Design review of the part built by this model. Coordinates are the model's own, in mm. A direction names the side the tool comes from. Give positions to 0.01 mm unless a question says otherwise; leave off trailing zeros. Order: outer loops, then holes, each group sorted by start corner. A loop starts at its lowest first (then second) coordinate and runs counter-clockwise, first axis right, second up. Notation, with made-up numbers: (2, 15) -> (55, 15) arc R24 cw to (55, 53) -> close; hole circle Ø1 at (13, 47.5). An arc over 180 degrees is marked (long way). One line per item, written item: value. Start each with the question number.
1) Consider section A-A (x = -70). State the section outline as (y, z) points.
2) For pin 1 (6 mm diameter, centred on x = 5.5, z = -14.5, fed in from +Y); pin 2 (1 mm diameter, centred on x = 141, z = -15, fed in from -Y); pin 3 (6 mm diameter, centred on x = -120.5, z = -28, fed in from +Y); pin 4 (19 mm diameter, centred on x = 80.5, y = -62.5, fed in from +Z), all flat-tipped, find the tip position at first contact; note any pin that passes through.
3) Consider section B-B (x = 41). State the section outline as (y, z) points.
4) Tool access review of faces 1 (the face through (3, -101, -2)), 2 (the face through (60.54, -112.55, 0.03)): name each direction out of +Z, -Z, +X, -X, +Y, -Y from which nothing blocks a thin tool from reaching the whole face with its end or side.
5) Wall thickness on line 1 along Y through (x, z) = (73, -0.55); line 2 along Z through (x, y) = (12, -181.5); line 3 along Y through (x, z) = (7, -0.4): over which ranges is each line inside the solid? List them lowest first. Write a range as from..to.
6) Consider section C-C (y = -219.5). State the section outline as (x, z) points, plus the area to 3 significant figures.
7) The part is to be moulded in two halves that separate along Y. For faces 3 (the face through (-177.15, -234.73, -30.62)), 4 (the face through (-2.544, -101.434, 0.028)), 5 (the face through (-180, -120.1, -1.7)), 6 (the face through (23.54, -112.55, 0.03)), say which applies: released by +Y, released by -Y, zero draft, split by the parting line, or undercut.
8) Consider section D-D (z = -19.5). State the section outline as (x, y) points.
from build123d import *

# Parameters (mm, degrees)
SALIENTE_EXTRUIR1_DEPTH = 180
CROQUIS3_R              = 12.450594948
CROQUIS3_R_2            = 15.7
CORTAR_EXTRUIR1_DEPTH   = 37.14486815
REDONDEO1_R             = 10


with BuildPart() as part:
    # Croquis1 → Saliente-Extruir1 (new body, symmetric)
    with BuildSketch(Plane(origin=(0, 0, 0), x_dir=(0, 0, -1), z_dir=(1, 0, 0))):
        with BuildLine():
            Line((-2, 0), (-2, -200))
            ThreePointArc((-2, -200), (-1.08655439, -204.592201188), (1.514718626, -208.485281374))
            Line((1.514718626, -208.485281374), (31.316441026, -238.287003774))
            Line((31.316441026, -238.287003774), (34.14486815, -235.458576649))
            Line((34.14486815, -235.458576649), (4.343145751, -205.656854249))
            ThreePointArc((4.343145751, -205.656854249), (2.60896374, -203.061467459), (2, -200))
            Line((2, -200), (2, 0))
            Line((2, 0), (-2, 0))
        make_face()
    extrude(amount=SALIENTE_EXTRUIR1_DEPTH, both=True)

    # Croquis3 → Cortar-Extruir1 (cut, through all)
    with BuildSketch(Plane.XY.offset(2)):
        with Locations((-70, -98)):
            Circle(CROQUIS3_R)
        with Locations((7, -77)):
            Circle(CROQUIS3_R_2)
        with Locations((-0.5, -117)):
            Circle(CROQUIS3_R_2)
        with Locations((36, -103)):
            Circle(CROQUIS3_R_2)
        with Locations((73, -103)):
            Circle(CROQUIS3_R_2)
        with Locations((110, -108)):
            Circle(CROQUIS3_R_2)
        with Locations((117.5, -68)):
            Circle(CROQUIS3_R_2)
        with Locations((80.5, -62.5)):
            Circle(CROQUIS3_R_2)
        with Locations((44, -62.5)):
            Circle(CROQUIS3_R_2)
    extrude(amount=-CORTAR_EXTRUIR1_DEPTH, mode=Mode.SUBTRACT)

    # Redondeo1
    redondeo1_edges = [part.edges().sort_by_distance(p)[0] for p in [
        (-180, 0, 0),
        (180, -236.872790212, -32.730654588),
        (180, 0, 0),
        (-180, -236.872790212, -32.730654588),
    ]]
    fillet(redondeo1_edges, radius=REDONDEO1_R)


solid = part.part
Checked values:
1. outline: (-238.29, -31.32) -> (-235.46, -34.14) -> (-205.66, -4.34) arc R8 cw to (-200, -2) -> (-110.45, -2) -> (-110.45, 2) -> (-200, 2) arc R12 ccw to (-208.49, -1.51) -> close; (-85.55, -2) -> (0, -2) -> (0, 2) -> (-85.55, 2) -> close
2. pin 1: stops at y = -212.81
2. pin 2: stops at y = -222.47
2. pin 3: stops at y = -226.31
2. pin 4: passes through
3. outline: (-238.29, -31.32) -> (-235.46, -34.14) -> (-205.66, -4.34) arc R8 cw to (-200, -2) -> (-117.88, -2) -> (-117.88, 2) -> (-200, 2) arc R12 ccw to (-208.49, -1.51) -> close; (-88.12, -2) -> (-77.91, -2) -> (-77.91, 2) -> (-88.12, 2) -> close; (-47.09, -2) -> (0, -2) -> (0, 2) -> (-47.09, 2) -> close
4. face 1: -Z, +X, -X, +Y
4. face 2: +Z, -Z
5. line 1: y = -207.4..-118.7, -87.3..-76.29, -48.71..0
5. line 2: z = -2..2
5. line 3: y = -207.2..-130.79, -103.21..-92.7, -61.3..0
6. outline: (-180, -18.19) -> (180, -18.19) -> (180, -12.53) -> (-180, -12.53) -> close
6. area: 2,040 mm^2
7. face 3: released by -Y
7. face 4: undercut
7. face 5: zero draft
7. face 6: undercut
8. outline: (-180, -226.47) -> (180, -226.47) -> (180, -220.81) -> (-180, -220.81) -> close
